For this review, take the finished solid that the model builds, in its own axes (mm). A direction names the side the tool comes from. Coordinates: 2 decimals unless noted, no trailing zeros. Write each loop counter-clockwise with the first axis right and the second up, starting at its lowest first coordinate (ties: lowest second). Pieces come first, ordered by that corner, then holes.
```python
from build123d import *

# Parameters (mm, degrees)
SKETCH1_R           = 3.5
BOSS_EXTRUDE2_DEPTH = 55
SKETCH7_W           = 68.999652055
SKETCH7_H           = 50.415620377
CUT_EXTRUDE5_DEPTH  = 13
SKETCH19_W          = 74.859412742
SKETCH19_H          = 60.725118028
CUT_EXTRUDE7_DEPTH  = 13


with BuildPart() as part:
    # Sketch1 → Boss-Extrude2 (new body)
    with BuildSketch(Plane(origin=(0, 0, 0), x_dir=(1, 0, 0), z_dir=(0, 1, 0))):
        with BuildLine():
            Line((-77.297393365, -66.943127962), (112.637979465, -57.343127962))
            add(Edge.make_bspline(
                [(112.637979465, -57.343127962), (125.082628436, -56.027724614), (133.287763268, -44.662014668), (142.702606635, -37.943127962)],
                knots=[0, 0, 0, 0, 1, 1, 1, 1], degree=3))
            Line((142.702606635, -37.943127962), (146.202606635, -37.943127962))
            Line((146.202606635, -37.943127962), (146.302606635, -37.943127962))
            ThreePointArc((146.302606635, -37.943127962), (150.120983253, -36.36150458), (151.702606635, -32.543127962))
            Line((151.702606635, -32.543127962), (151.702606635, 23.656872038))
            ThreePointArc((151.702606635, 23.656872038), (150.120983253, 27.475248656), (146.302606635, 29.056872038))
            Line((146.302606635, 29.056872038), (146.202606635, 29.056872038))
            Line((146.202606635, 29.056872038), (142.702606635, 29.056872038))
            add(Edge.make_bspline(
                [(112.637979465, 48.456872038), (125.082628436, 47.14146869), (133.287763268, 35.775758744), (142.702606635, 29.056872038)],
                knots=[0, 0, 0, 0, 1, 1, 1, 1], degree=3))
            Line((112.637979465, 48.456872038), (-77.297393365, 58.056872038))
            add(Edge.make_bspline(
                [(-77.297393365, 58.056872038), (-97.47829568, 56.558543187), (-92.669908534, 31.299380259), (-112.297393365, 29.056872038)],
                knots=[0, 0, 0, 0, 1, 1, 1, 1], degree=3))
            Line((-112.297393365, 29.056872038), (-115.797393365, 29.056872038))
            Line((-115.797393365, 29.056872038), (-115.897393365, 29.056872038))
            ThreePointArc((-115.897393365, 29.056872038), (-119.715769983, 27.475248656), (-121.297393365, 23.656872038))
            Line((-121.297393365, 23.656872038), (-121.297393365, -32.543127962))
            ThreePointArc((-121.297393365, -32.543127962), (-119.715769983, -36.36150458), (-115.897393365, -37.943127962))
            Line((-115.897393365, -37.943127962), (-115.797393365, -37.943127962))
            Line((-115.797393365, -37.943127962), (-112.297393365, -37.943127962))
            add(Edge.make_bspline(
                [(-77.297393365, -66.943127962), (-97.47829568, -65.444799111), (-92.669908534, -40.185636183), (-112.297393365, -37.943127962)],
                knots=[0, 0, 0, 0, 1, 1, 1, 1], degree=3))
        make_face()
        with Locations((-112.297393365, 20.556872038)):
            Circle(SKETCH1_R, mode=Mode.SUBTRACT)
        with Locations((-112.297393365, -29.443127962)):
            Circle(SKETCH1_R, mode=Mode.SUBTRACT)
        with Locations((142.702606635, -29.443127962)):
            Circle(SKETCH1_R, mode=Mode.SUBTRACT)
        with Locations((142.702606635, 20.556872038)):
            Circle(SKETCH1_R, mode=Mode.SUBTRACT)
    extrude(amount=-BOSS_EXTRUDE2_DEPTH)

    # Sketch7 → Cut-Extrude5 (cut)
    with BuildSketch(Plane.ZY.offset(121.297393365)):
        with Locations((4.333112833, -30.707810189)):
            Rectangle(SKETCH7_W, SKETCH7_H)
    extrude(amount=-CUT_EXTRUDE5_DEPTH, mode=Mode.SUBTRACT)

    # Sketch19 → Cut-Extrude7 (cut)
    with BuildSketch(Plane(origin=(151.702606635, 0, 0), x_dir=(0, 0, -1), z_dir=(1, 0, 0))):
        with Locations((-5.097493458, -35.862559014)):
            Rectangle(SKETCH19_W, SKETCH19_H)
    extrude(amount=-CUT_EXTRUDE7_DEPTH, mode=Mode.SUBTRACT)


solid = part.part
```
Q1. Clearance check with flat-ended pins moving along their axes: pin 1 Ø5 at (x, y) = (111.5, -8) entering from +Z; pin 2 Ø1.5 at (y, z) = (-33.5, 32) entering from -X; pin 3 Ø1.5 at (y, z) = (-37, 15.5) entering from +X; pin 4 Ø6.5 at (x, z) = (142.7, -20.56) entering from +Y. State where each tip first meets the part, or that it passes through.
Ans:
pin 1: stops at z = 57.53
pin 2: stops at x = -108.3
pin 3: stops at x = 138.7
pin 4: passes through
Q2. Draft analysis for pull direction X (two halves, no side actions). For faces 1 (the cylindrical face through (145.936, -2.712, -19.216)), 2 (the flat face through (19, -27.12, -53.19)), 3 (the flat face through (-108.297, -30, 4)), state which applies: +X half, -X half, draft (parallel to the pull), parting line (faces both ways), or undercut.
Ans:
face 1: undercut
face 2: +X half
face 3: -X half
Q3. Add section C-C (x = -49). State the section outline as (y, z) points, then the cut area to 3 significant figures.
Ans:
outline: (-55, -56.63) - (0, -56.63) - (0, 65.51) - (-55, 65.51) - close
area: 6,720 mm2
Q4. Add section A-A (z = -8). State the section outline as (x, y) points, then the cut area to 3 significant figures.
Ans:
outline: (-121.3, -5.5) - (-108.3, -5.5) - (-108.3, -55) - (138.7, -55) - (138.7, -5.5) - (151.7, -5.5) - (151.7, 0) - (-121.3, 0) - close
area: 13,700 mm2
Q5. Add section B-B (x = 96.5). State the section outline as (y, z) points.
Ans:
outline: (-55, -49.27) - (0, -49.27) - (0, 58.16) - (-55, 58.16) - close
Q6. Tool access review of faces 4 (the flat face through (-115, -5.5, 4)), 5 (the cylindrical face through (145.936, -2.712, 30.784)), 6 (the flat face through (145, -5.5, 5)): name each direction out of +Z, -Z, +X, -X, +Y, -Y from which nothing blocks a thin tool from reaching the whole face with its end or side.
Ans:
face 4: +Z, -Z, -X, -Y
face 5: +Y, -Y
face 6: +Z, -Z, +X, -Y
Q7. For probe 1 along X at (y, z) = (-8, -19); probe 2 along Z at (x, y) = (-20, -31.5); probe 3 along Z at (x, y) = (-12, -27.5), list the stretches that pass through material, from the lowest coordinate up.
Ans:
probe 1: x = -108.3 to 138.7
probe 2: z = -55.16 to 64.05
probe 3: z = -54.76 to 63.64
